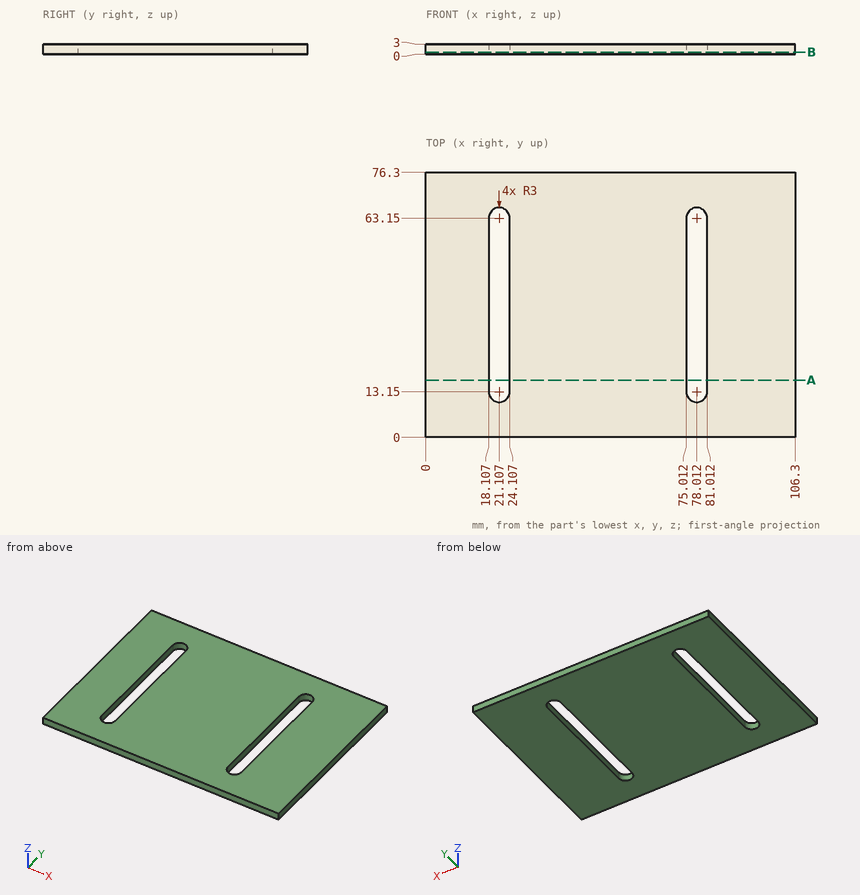
The figure shows three views and two pictorial views of one solid part (mm, origin at its lowest corner). Answer the questions. Give positions to 0.01 mm unless a question says otherwise; leave off trailing zeros. Write each loop counter-clockwise with the first axis right and the second up, starting at its lowest first coordinate (ties: lowest second). Pieces come first, ordered by that corner, then holes. Notation, with made-up numbers: (-18, -8) - (-6, -8) arc R15 ccw to (-6, 5) - close; hole circle Ø10 at (-14, 37.5). An arc over 180 degrees is marked (long way). Return JSON: item names as keys, results as strings.
Q1. A cutting plane is placed at B-B, the plane z = 0.65. Determine the outline of the cut face in (x, y).
Reply:
{"outline": "(0, 0) - (106.3, 0) - (106.3, 76.3) - (0, 76.3) - close; hole (18.11, 13.15) arc R3 ccw to (24.11, 13.15) - (24.11, 63.15) arc R3 ccw to (18.11, 63.15) - close; hole (75.01, 13.15) arc R3 ccw to (81.01, 13.15) - (81.01, 63.15) arc R3 ccw to (75.01, 63.15) - close"}
Q2. A cutting plane is placed at A-A, the plane y = 16.5. Determine the outline of the cut face in (x, z), and give its area (3 significant figures).
Reply:
{"outline": "(0, 0) - (18.11, 0) - (18.11, 3) - (0, 3) - close; (24.11, 0) - (75.01, 0) - (75.01, 3) - (24.11, 3) - close; (81.01, 0) - (106.3, 0) - (106.3, 3) - (81.01, 3) - close", "area": "283 mm²"}
Q3. Consider line 1 along X through (y, z) = (54.5, 0.4); line 2 along X through (y, z) = (12, 1.6). Determine where each line is inside the solid, lowest interval first. Write a range as [from, to].
Reply:
{"line 1": "[0, 18.11], [24.11, 75.01], [81.01, 106.3]", "line 2": "[0, 18.34], [23.88, 75.24], [80.78, 106.3]"}
